Source: CAD feature listing. Evaluate the final solid. Frame: model axes, mm. Face numbers are marked on the shaded views. A direction names the side the tool comes from. Round coordinates to 2 decimals unless told otherwise and drop trailing zeros. Order: outer loops, then holes, each group sorted by start corner. A loop starts at its lowest first (then second) coordinate and runs counter-clockwise, first axis right, second up. Notation, with made-up numbers: (-22, 76) -> (-5, 76) arc R27 ccw to (-5, 115) -> close; hole circle Ø7 at (13, -18.75). An arc over 180 degrees is marked (long way). Answer as CSV lines item,"result". Start each with the question number.
(1) Section query B-B (x = 86). Output: boundary loops of the cut face in (y, z) (3 decimals), plus the area to 3 significant figures.
(2) Section query D-D (y = 3.25). Output: boundary loops of the cut face in (x, z), plus the area to 3 significant figures.
(3) Pull-direction query (X, two-part tool) for the marked faces 1, 2, 3 and 4; classes: +X half, -X half, draft (parallel to the pull), parting line (faces both ways), or undercut.
(4) Set-up query: the marked faces 5, 6, 7 and 8. Return all of +Z, -Z, +X, -X, +Y, -Y with unobstructed straight access to the full face (end or side cutting, diameter ignored); none if empty.
(5) Line query: line 1 along X through (y, z) = (1.75, -16); line 2 along X through (y, z) = (6.5, -40); line 3 along X through (y, z) = (-1.75, -16). Output: solid intervals per line, ascending. Write a range as from..to.
(6) Section query C-C (z = -16). Output: boundary loops of the cut face in (x, y) (3 decimals).
(7) Contact query for flat-ended pins moving along their axis: P1, Ø10.5, axis at x = 129, y = 6, coming from the +Z side; P2, Ø1.5, axis at x = 176, z = -46, coming from the +Y side; P3, Ø4.5, axis at x = 167.79, z = -57.93, coming from the -Y side. Output: stop coordinate, or through.
(8) Section query A-A (z = -28.5). Output: boundary loops of the cut face in (x, y) (3 decimals), plus the area to 3 significant figures.
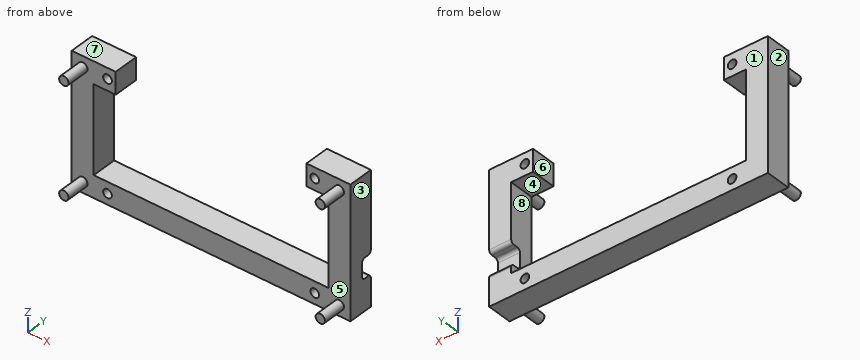
```python
from build123d import *

# Parameters (mm, degrees)
SKETCH1_R           = 1.651
BOSS_EXTRUDE1_DEPTH = 9.525
SKETCH2_W           = 7.62
SKETCH2_H           = 4.099575227
CUT_EXTRUDE7_DEPTH  = 8.89
FILLET2_R           = 1.27
SKETCH3_R           = 1.778
BOSS_EXTRUDE3_DEPTH = 8.89


with BuildPart() as part:
    # Sketch1 → Boss-Extrude1 (new body)
    with BuildSketch(Plane(origin=(0, 0, 0), x_dir=(1, 0, 0), z_dir=(0, 1, 0))):
        Polygon((75.155177047, 61.997896552), (75.155177047, 11.997896552), (91.919177047, 11.997896552), (91.919177047, 20.379896552), (83.537177047, 20.379896552), (83.537177047, 53.615896552), (173.037829354, 53.615896552), (173.037829354, 20.379896552), (164.655829354, 20.379896552), (164.655829354, 11.997896552), (181.419829354, 11.997896552), (181.419829354, 61.997896552), align=None)
        with Locations(Location((88.7874552, 16.064784874, 0), (0, 0, 90))):
            Circle(SKETCH1_R, mode=Mode.SUBTRACT)
        with Locations(Location((167.7875512, 57.93100823, 0), (0, 0, 90))):
            Circle(SKETCH1_R, mode=Mode.SUBTRACT)
        with Locations(Location((88.7874552, 57.93100823, 0), (0, 0, 90))):
            Circle(SKETCH1_R, mode=Mode.SUBTRACT)
        with Locations(Location((167.7875512, 16.064784874, 0), (0, 0, 90))):
            Circle(SKETCH1_R, mode=Mode.SUBTRACT)
    extrude(amount=BOSS_EXTRUDE1_DEPTH)

    # Sketch2 → Cut-Extrude7 (cut)
    with BuildSketch(Plane(origin=(181.419829354, 0, 0), x_dir=(0, 0, -1), z_dir=(1, 0, 0))):
        with Locations((46.287896552, 7.475212387)):
            Rectangle(SKETCH2_W, SKETCH2_H)
    extrude(amount=-CUT_EXTRUDE7_DEPTH, mode=Mode.SUBTRACT)

    # Fillet2
    fillet2_edges = [part.edges().sort_by_distance(p)[0] for p in [
        (177.228829354, 9.525, -42.477896552),
        (177.228829354, 9.525, -50.097896552),
        (177.228829354, 5.425424773, -50.097896552),
        (177.228829354, 5.425424773, -42.477896552),
    ]]
    fillet(fillet2_edges, radius=FILLET2_R)

    # Sketch3 → Boss-Extrude3 (add)
    with BuildSketch(Plane.XZ):
        with Locations(Location((79.3894552, -16.064784874, 0), (0, 0, 90))):
            Circle(SKETCH3_R)
        with Locations(Location((177.1855512, -16.064784874, 0), (0, 0, 90))):
            Circle(SKETCH3_R)
        with Locations(Location((79.3894552, -57.93100823, 0), (0, 0, 90))):
            Circle(SKETCH3_R)
        with Locations(Location((177.1855512, -57.93100823, 0), (0, 0, 90))):
            Circle(SKETCH3_R)
    extrude(amount=BOSS_EXTRUDE3_DEPTH)


solid = part.part
```
Answer block:
1,outline,"(0, -61.998) -> (9.525, -61.998) -> (9.525, -53.616) -> (0, -53.616) -> close; (0, -20.38) -> (9.525, -20.38) -> (9.525, -11.998) -> (0, -11.998) -> close"
1,area,"160 mm2"
2,outline,"(75.16, -62) -> (181.42, -62) -> (181.42, -12) -> (164.66, -12) -> (164.66, -20.38) -> (173.04, -20.38) -> (173.04, -53.62) -> (83.54, -53.62) -> (83.54, -20.38) -> (91.92, -20.38) -> (91.92, -12) -> (75.16, -12) -> close; hole circle Ø3.3 at (88.79, -57.93); hole circle Ø3.3 at (88.79, -16.06); hole circle Ø3.3 at (167.79, -57.93); hole circle Ø3.3 at (167.79, -16.06)"
2,area,"1,690 mm2"
3,face 1,"draft"
3,face 2,"-X half"
3,face 3,"+X half"
3,face 4,"undercut"
4,face 5,"-Y"
4,face 6,"+Z, +Y, -Y"
4,face 7,"+Z, +X, -X, +Y, -Y"
4,face 8,"+Y, -Y"
5,line 1,"75.16..87.14, 90.44..91.92, 164.66..166.14, 169.44..181.42"
5,line 2,"75.16..83.54, 173.04..181.42"
5,line 3,"77.61..81.17, 175.41..178.96"
6,outline,"(75.155, 0) -> (77.613, 0) -> (77.613, -8.89) -> (81.166, -8.89) -> (81.166, 0) -> (87.138, 0) -> (87.138, 9.525) -> (75.155, 9.525) -> close; (90.437, 0) -> (91.919, 0) -> (91.919, 9.525) -> (90.437, 9.525) -> close; (164.656, 0) -> (166.138, 0) -> (166.138, 9.525) -> (164.656, 9.525) -> close; (169.437, 0) -> (175.409, 0) -> (175.409, -8.89) -> (178.962, -8.89) -> (178.962, 0) -> (181.42, 0) -> (181.42, 9.525) -> (169.437, 9.525) -> close"
7,P1,"z = -53.62"
7,P2,"y = 5.43"
7,P3,"y = 0"
8,outline,"(75.155, 0) -> (83.537, 0) -> (83.537, 9.525) -> (75.155, 9.525) -> close; (173.038, 0) -> (181.42, 0) -> (181.42, 9.525) -> (173.038, 9.525) -> close"
8,area,"160 mm2"
